Read the model definition and answer for the solid it produces. Units are mm, in the model's axes. A direction names the side the tool comes from. Round coordinates to 2 decimals unless told otherwise and drop trailing zeros. Order: outer loops, then holes, each group sorted by start corner. A loop starts at its lowest first (then second) coordinate and runs counter-clockwise, first axis right, second up. Notation, with made-up numbers: (13, -23.75) - (19, -23.75) arc R9 ccw to (19, -16.75) - close; hole circle Ø2 at (68, -8). An arc over 180 degrees is marked (long way). Put each result on its own line as item: value. Start each with the question number.
Q1. Section B-B on y = -7.5 is taken. Give the vertices of the cut face in (x, z), then the cut area to 3 significant figures.
Q2. Find the intervals of material crossed by line 1 along X through (y, z) = (7.5, 1.3); line 2 along X through (y, z) = (-7.5, 1.15); line 3 along X through (y, z) = (8.25, 6.75), in increasing order. Write a range as from..to.
Q3. Which of the six approach directions +Z, -Z, +X, -X, +Y, -Y give full straight-line access (tool end or side, diameter ignored) to faces 4 (the face through (12.3, 10.45, 5.77)), 5 (the face through (16.369, 9.286, 1.775))?
Q4. Section A-A on x = -15 is taken. Give the vertices of the cut face in (y, z).
Q5. Each of these flat-tipped pins is pushed along its axis until it touches: pin 1 Ø6 at (x, y) = (15, 7.5) entering from +Z; pin 2 Ø6 at (x, y) = (0, 0) entering from +Z; pin 3 Ø1.8 at (x, y) = (0, 9) entering from +Z. Where does it stop, or does it pass through?
Q6. Section C-C on z = 6.5 is taken. Give the vertices of the cut face in (x, y).
Q7. Section D-D on z = 0.75 is taken. Give the vertices of the cut face in (x, y), then the cut area to 3 significant figures.
Q8. For a pull along Y with two mould halves and no side action, classify faces 1 (the face through (0, 12.5, 4)), 2 (the face through (20, 0, 4)), 3 (the face through (-12.804, -7.012, 1.775)) as pulls with the +Y half, pulls with the -Y half, needs draft (parallel to the pull), parting line crosses it, or undercut.
Autodesk Inventor part; units mm, degrees
ref_plane "YZ Plane" through (0, 0, 0) normal (1, 0, 0) x (0, 1, 0)
ref_plane "XZ Plane" through (0, 0, 0) normal (0, 1, 0) x (-1, 0, 0)
ref_plane "XY Plane" through (0, 0, 0) normal (0, 0, 1) x (1, 0, 0)
sketch "Skizze1" plane through (0, 0, 0) normal (0, 0, 1) x (1, 0, 0)
  line L0 (-20, 12.5) -> (20, 12.5)
  line L1 (20, 12.5) -> (20, -12.5)
  line L2 (20, -12.5) -> (-20, -12.5)
  line L3 (-20, -12.5) -> (-20, 12.5)
  line L4 (-28, 0) -> (28, 0)
  line L5 (0, -17.5) -> (0, 17.5)
  point P0 (0, 0)
  dimension "d0" = 40
  dimension "d1" = 25
extrude "Extrusion1" add sketch "Skizze1" along normal blind 8
sketch "Skizze2" plane through (0, 0, 8) normal (0, 0, 1) x (1, 0, 0)
  line L0 (-28, 0) -> (28, 0)
  line L1 (0, -17.5) -> (0, 17.5)
  line L2 (-15, 7.5) -> (15, 7.5)
  line L3 (15, 7.5) -> (15, -7.5)
  line L4 (15, -7.5) -> (-15, -7.5)
  line L5 (-15, -7.5) -> (-15, 7.5)
  point P0 (0, 0)
  dimension "d4" = 15
  dimension "d5" = 30
hole "Bohrung1" at (-15, -7.5, 8) at (15, 7.5, 8) direction (0, 0, -1) diameter 4.5 end through all counterbore diameter 8 counterbore depth 4.4
sketch "Skizze3" plane through (0, 0, 8) normal (0, 0, 1) x (1, 0, 0)
  point P0 (0, 0)
  point P1 (0, 0)
hole "Bohrung2" at (0, 0, 8) direction (0, 0, -1) diameter 3 end through all
hole "Bohrung3" at (0, 0, 0) direction (0, 0, 1) diameter 6.6 end through all countersink diameter 12.4 countersink angle 90
sketch "Skizze4" plane through (0, 0, 8) normal (0, 0, 1) x (1, 0, 0)
  line L0 (-28, 0) -> (28, 0)
  line L1 (0, -17.5) -> (0, 17.5)
  point P0 (0, 9)
  dimension "d29" = 9
hole "Bohrung4" at (0, 9, 8) direction (0, 0, -1) diameter 2.2 depth 5 tip angle 118
properties part number "13_0204_074"
Findings:
1. outline: (-20, 0) - (-17.25, 0) - (-17.25, 3.6) - (-19, 3.6) - (-19, 8) - (-20, 8) - close; (-12.75, 0) - (20, 0) - (20, 8) - (-11, 8) - (-11, 3.6) - (-12.75, 3.6) - close
1. area: 269 mm2
2. line 1: -20..12.75, 17.25..20
2. line 2: -20..-17.25, -12.75..20
2. line 3: -20..-0.8, 0.8..11.07, 18.93..20
3. face 4: +Z
3. face 5: +Z, -Z
4. outline: (-12.5, 0) - (-9.75, 0) - (-9.75, 3.6) - (-11.5, 3.6) - (-11.5, 8) - (-12.5, 8) - close; (-5.25, 0) - (12.5, 0) - (12.5, 8) - (-3.5, 8) - (-3.5, 3.6) - (-5.25, 3.6) - close
5. pin 1: z = 3.6
5. pin 2: through
5. pin 3: z = 2.88
6. outline: (-20, -12.5) - (20, -12.5) - (20, 12.5) - (-20, 12.5) - close; hole circle Ø8 at (-15, -7.5); hole circle Ø6.6 at (0, 0); hole circle Ø2.2 at (0, 9); hole circle Ø8 at (15, 7.5)
7. outline: (-20, -12.5) - (20, -12.5) - (20, 12.5) - (-20, 12.5) - close; hole circle Ø4.5 at (-15, -7.5); hole circle Ø10.9 at (0, 0); hole circle Ø4.5 at (15, 7.5)
7. area: 875 mm2
8. face 1: pulls with the +Y half
8. face 2: needs draft
8. face 3: undercut
